CAD build for the part. Positions are in the model's coordinates, mm. A direction names the side the tool comes from. Round coordinates to 2 decimals unless told otherwise and drop trailing zeros. Loops run counter-clockwise (first coordinate to the right, second up) from the corner with the lowest first, then second, coordinate; pieces in that order, holes last. Notation, with made-up numbers: M 19,11.5 L 34,11.5 A26 cw 34,34.5 Z; hole C 67.5,38.25 d3. An arc over 180 degrees is marked long. Use one line per item in the form item = value.
from build123d import *

# Parameters (mm, degrees)
SKETCH3_R           = 3.175
SKETCH3_R_2         = 1.905
BOSS_EXTRUDE1_DEPTH = 5.08


with BuildPart() as part:
    # Sketch1 → Revolve1 (revolve)
    with BuildSketch(Plane.XY, mode=Mode.PRIVATE) as revolve1_sk:
        Polygon((-38.1, -2.54), (0, -2.54), (0, 0), (-50.8, 0), (-50.8, -5.08), (-38.1, -5.08), align=None)
    revolve(revolve1_sk.sketch.rotate(Axis((0, 4.567685351, 0), (0, -1, 0)), 270), axis=Axis((0, 4.567685351, 0), (0, -1, 0)))

    # Sketch3 → Boss-Extrude1 (add)
    # profile 1 of 3: a face of its own
    with BuildSketch(Plane(origin=(0, 0, 0), x_dir=(1, 0, 0), z_dir=(0, 1, 0))):
        with Locations(Location((-38.1, 0, 0), (0, 0, 270))):
            Circle(SKETCH3_R)
        with Locations(Location((-38.1, 0, 0), (0, 0, 270))):
            Circle(SKETCH3_R_2, mode=Mode.SUBTRACT)
    # profile 2 of 3: a face of its own
    with BuildSketch(Plane(origin=(0, 0, 0), x_dir=(1, 0, 0), z_dir=(0, 1, 0))):
        with Locations(Location((19.05, 32.995567884, 0), (0, 0, 270))):
            Circle(SKETCH3_R)
        with Locations(Location((19.05, 32.995567884, 0), (0, 0, 270))):
            Circle(SKETCH3_R_2, mode=Mode.SUBTRACT)
    # profile 3 of 3: a face of its own
    with BuildSketch(Plane(origin=(0, 0, 0), x_dir=(1, 0, 0), z_dir=(0, 1, 0))):
        with Locations(Location((19.05, -32.995567884, 0), (0, 0, 270))):
            Circle(SKETCH3_R)
        with Locations(Location((19.05, -32.995567884, 0), (0, 0, 270))):
            Circle(SKETCH3_R_2, mode=Mode.SUBTRACT)
    extrude(amount=BOSS_EXTRUDE1_DEPTH)


solid = part.part
1. Cut at B-B on z = 0. Write the cut outline in (x, y) (3 decimals).
Completed:
outline = M -50.8,-5.08 L -38.1,-5.08 L -38.1,-2.54 L 38.1,-2.54 L 38.1,-5.08 L 50.8,-5.08 L 50.8,0 L -34.925,0 L -34.925,5.08 L -36.195,5.08 L -36.195,0 L -40.005,0 L -40.005,5.08 L -41.275,5.08 L -41.275,0 L -50.8,0 Z
2. Cut at D-D on x = 12.5. Write the cut outline in (y, z), and give its area (3 significant figures).
Completed:
outline = M -5.08,-49.24 L 0,-49.24 L 0,49.24 L -5.08,49.24 L -5.08,35.99 L -2.54,35.99 L -2.54,-35.99 L -5.08,-35.99 Z
area = 317 mm2
3. Cut at A-A on y = 3.5. Write the cut outline in (x, z) (3 decimals), and give its area (3 significant figures).
Completed:
outline = C -38.1,0 d6.35; C 19.05,-32.996 d6.35; C 19.05,32.996 d6.35; hole C -38.1,0 d3.81; hole C 19.05,-32.996 d3.81; hole C 19.05,32.996 d3.81
area = 60.8 mm2
4. Tool access for faces 1 (the face through (19, 0, 33)), 2 (the face through (30.911, -2.576, -40.313)), 3 (the face through (23.183, -3.792, -30.235)): list every direction of +Z, -Z, +X, -X, +Y, -Y with a clear straight run to the whole face (end or side of a thin tool).
Completed:
face_1 = +Y
face_2 = +Y, -Y
face_3 = -Y
5. Cut at C-C on x = 0. Write the cut outline in (y, z), and give its area (3 significant figures).
Completed:
outline = M -5.08,-50.8 L 0,-50.8 L 0,50.8 L -5.08,50.8 L -5.08,38.1 L -2.54,38.1 L -2.54,-38.1 L -5.08,-38.1 Z
area = 323 mm2
6. Pull direction X, two halves, no side cores. Call faces 4 (the face through (17.891, 2.504, -34.507)), 5 (the face through (-40.2, 5.08, 0)), 6 (the face through (17.1, 2.5, -35.5)): +X half, -X half, draft (parallel to the pull), parting line (faces both ways), or undercut.
Completed:
face_4 = undercut
face_5 = draft
face_6 = parting line
7. Drop flat-ended pins along their axis: P1, Ø5, axis at y = -2.5, z = -26, coming from the +X side; P2, Ø10, axis at x = -7.5, z = -17, coming from the +Y side; P3, Ø2, axis at x = 18, y = 3.5, coming from the -Z side. Give the stop position or say it passes through.
Completed:
P1 = 45.04
P2 = 0
P3 = -36.17
8. Probe line 1 along Y through (x, z) = (25.5, -43); line 2 along X through (y, z) = (-4.45, 0); line 3 along X through (y, z) = (-4, -7). List the from-to ranges inside material, lowest first. Write a range as from..to.
Completed:
line_1 = -5.08..0
line_2 = -50.8..-38.1, 38.1..50.8
line_3 = -50.32..-37.45, 37.45..50.32
